```python
from build123d import *

# Parameters (mm, degrees)
SKETCH1_W           = 360
SKETCH1_H           = 102
BOSS_EXTRUDE1_DEPTH = 2
SKETCH2_W           = 36
SKETCH2_H           = 51
SKETCH2_W_2         = 113
SKETCH2_H_2         = 35
CUT_EXTRUDE1_DEPTH  = 10
SKETCH3_W           = 57
SKETCH3_H           = 28
CUT_EXTRUDE2_DEPTH  = 10


with BuildPart() as part:
    # Sketch1 → Boss-Extrude1 (new body)
    with BuildSketch(Plane(origin=(0, 0, 0), x_dir=(0, 0, -1), z_dir=(1, 0, 0))):
        with Locations((62.608695652, 70.304347826)):
            Rectangle(SKETCH1_W, SKETCH1_H)
    extrude(amount=BOSS_EXTRUDE1_DEPTH)

    # Sketch2 → Cut-Extrude1 (cut)
    with BuildSketch(Plane.ZY):
        with Locations((56.914343826, 44.804347826)):
            Rectangle(SKETCH2_W, SKETCH2_H)
        with Locations((-69.366260537, 67.630807185)):
            Rectangle(SKETCH2_W_2, SKETCH2_H_2)
    extrude(amount=-CUT_EXTRUDE1_DEPTH, mode=Mode.SUBTRACT)

    # Sketch3 → Cut-Extrude2 (cut)
    with BuildSketch(Plane.ZY):
        with Locations((-194.333824882, 85.510777566)):
            Rectangle(SKETCH3_W, SKETCH3_H)
    extrude(amount=-CUT_EXTRUDE2_DEPTH, mode=Mode.SUBTRACT)


solid = part.part
```
The model under review builds one solid part; all positions refer to its coordinate system, in mm. Round coordinates to 2 decimals unless told otherwise and drop trailing zeros. Loops run counter-clockwise (first coordinate to the right, second up) from the corner with the lowest first, then second, coordinate; pieces in that order, holes last. Notation, with made-up numbers: (21.5, 59.25) -> (64.5, 59.25) arc R15 ccw to (64.5, 72.25) -> close; hole circle Ø6 at (-15, -25.5). An arc over 180 degrees is marked (long way). Answer as a JSON object with one key per item and string values. Group by question number.
1) For line 1 (Z direction, x = 0.65, y = 70); line 2 (Z direction, x = 0.55, y = 73.5); line 3 (Y direction, x = 0.75, z = -22), list the stretches that pass through material, from the lowest coordinate up. Write a range as [from, to].
2) We need section C-C on x = 1.2. Write out the cut boundary in (y, z).
3) We need section B-B on y = 90.5. Write out the cut boundary in (x, z), then the cut area to 3 significant figures.
4) For pin 1 Ø6 at (y, z) = (59.5, 70.5) entering from +X; pin 2 Ø10 at (y, z) = (42, 42) entering from -X; pin 3 Ø0.6 at (x, z) = (1, 58) entering from -Y, all flat-tipped, find the tip position at first contact; note any pin that passes through.
5) We need section A-A on z = -208. Write out the cut boundary in (x, y), then the cut area to 3 significant figures.
6) We need section D-D on z = 63. Write out the cut boundary in (x, y), then the cut area to 3 significant figures.
Result set:
{
 "1": {"line 1": "[-242.61, -125.87], [-12.87, 38.91], [74.91, 117.39]", "line 2": "[-242.61, -222.83], [-165.83, -125.87], [-12.87, 117.39]", "line 3": "[19.3, 50.13], [85.13, 121.3]"},
 "2": {"outline": "(19.3, -242.61) -> (121.3, -242.61) -> (121.3, 117.39) -> (19.3, 117.39) -> (19.3, 74.91) -> (70.3, 74.91) -> (70.3, 38.91) -> (19.3, 38.91) -> close; hole (50.13, -125.87) -> (85.13, -125.87) -> (85.13, -12.87) -> (50.13, -12.87) -> close; hole (71.51, -222.83) -> (99.51, -222.83) -> (99.51, -165.83) -> (71.51, -165.83) -> close"},
 "3": {"outline": "(0, -242.61) -> (2, -242.61) -> (2, -222.83) -> (0, -222.83) -> close; (0, -165.83) -> (2, -165.83) -> (2, 117.39) -> (0, 117.39) -> close", "area": "606 mm²"},
 "4": {"pin 1": "through", "pin 2": "x = 0", "pin 3": "y = 70.3"},
 "5": {"outline": "(0, 19.3) -> (2, 19.3) -> (2, 71.51) -> (0, 71.51) -> close; (0, 99.51) -> (2, 99.51) -> (2, 121.3) -> (0, 121.3) -> close", "area": "148 mm²"},
 "6": {"outline": "(0, 70.3) -> (2, 70.3) -> (2, 121.3) -> (0, 121.3) -> close", "area": "102 mm²"}
}
